from build123d import *

# Parameters (mm, degrees)
ESBO_O2_R       = 1.6
EXTRUS_O1_DEPTH = 30


with BuildPart() as part:
    # Varredura1: sweep along a path in Esboço1
    with BuildLine(Plane.XY) as varredura1_path:
        Line((1.65, 166.275006099), (1.65, 16.275006099))
        Line((1.65, 16.275006099), (7.405965146, 3.2805))
        ThreePointArc((7.405965146, 3.2805), (0, -8.1), (-7.405965146, 3.2805))
        Line((-7.405965146, 3.2805), (-1.65, 16.275006099))
        Line((-1.65, 16.275006099), (-1.65, 51.275006099))
    # Esboço2 → Varredura1 (sweep)
    with BuildSketch(Plane(origin=(1.65, 166.275006099, 0), x_dir=(1, 0, 0), z_dir=(0, -1, 0))):
        Circle(ESBO_O2_R)
    sweep(path=varredura1_path.line, transition=Transition.RIGHT)

    # Esboço4 → Extrusão1 (add)
    with BuildSketch(Plane(origin=(0, 20, 0), x_dir=(-1, 0, 0), z_dir=(0, 1, 0))):
        Polygon((-5.773502692, 0), (-2.886751346, -5), (2.886751346, -5), (5.773502692, 0), (2.886751346, 5), (-2.886751346, 5), align=None)
    extrude(amount=EXTRUS_O1_DEPTH)


solid = part.part
Read the model definition and answer for the solid it produces. Units are mm, in the model's axes. A direction names the side the tool comes from. Coordinates: 2 decimals unless noted, no trailing zeros. Loops run counter-clockwise (first coordinate to the right, second up) from the corner with the lowest first, then second, coordinate; pieces in that order, holes last.
Q1. Consider probe 1 along Y at (x, z) = (-4.75, -0.5); probe 2 along Z at (x, y) = (1.75, 101); probe 3 along Y at (x, z) = (-4.5, 1). Determine where each line is inside the solid, lowest interval first.
Q2. The part is cut by section B-B on z = -3.25. Write down the section's boundary in (x, y).
Q3. The part is cut by section A-A on y = 95. Write down the section's boundary in (x, z), and give its area (3 significant figures).
Q4. The mould has two halves that part along Y. Classify faces 5 (the face through (0.4, 17.9, -1)), 6 (the face through (-4.101, 9.885, -1.562)), 7 (the face through (2, 166.275, 0)), 8 (the face through (-4.31, 34.79, -2.535)): +Y half, -Y half, draft (parallel to the pull), parting line (faces both ways), or undercut.
Q5. Each of these flat-tipped pins is pushed along its axis until it touches: pin 1 Ø6 at (x, z) = (3.5, 1.5) entering from -Y; pin 2 Ø5 at (x, z) = (-2.5, 0) entering from +Y (3 decimals); pin 3 Ø5 at (y, z) = (116.5, 0) entering from -X. Where does it stop, or does it pass through?
Q6. Which of the six approach directions +Z, -Z, +X, -X, +Y, -Y give full straight-line access (tool end or side, diameter ignored) to faces 1 (the face through (4.31, 34.79, 2.535)), 2 (the face through (-0.47, 18, 1.08)), 3 (the face through (4.35, 34.79, -2.465)), 4 (the face through (-4.35, 34.79, 2.465))?
Results below:
1. probe 1: y = -8.37 to -4.55, 5.52 to 13.03, 20 to 50
1. probe 2: z = -1.6 to 1.6
1. probe 3: y = -8.19 to -5.17, 6.76 to 12.92, 20 to 50
2. outline: (-3.9, 20) - (3.9, 20) - (3.9, 50) - (-3.9, 50) - close
3. outline: circle Ø3.2 at (1.65, 0)
3. area: 8.04 mm2
4. face 5: undercut
4. face 6: undercut
4. face 7: +Y half
4. face 8: draft
5. pin 1: stops at y = -9.66
5. pin 2: stops at y = 51.275
5. pin 3: stops at x = 0.05
6. face 1: +Z, +X, +Y
6. face 2: none
6. face 3: -Z, +X, +Y
6. face 4: +Z, -X, +Y
